from build123d import *

# Parameters (mm, degrees)
SKETCH_1_W          = 13
SKETCH_1_H          = 2.1
SKETCH_1_W_2        = 8
EXTRUDE_3_DEPTH     = 2
SKETCH_2_W          = 6.1
SKETCH_2_H          = 2.1
CUT_EXTRUDE_1_DEPTH = 2
SKETCH_12_W         = 13
SKETCH_12_H         = 2.1
EXTRUDE_9_DEPTH     = 2
SKETCH_13_R         = 1.7
EXTRUDE_10_DEPTH    = 2
SKETCH_3_W          = 16.8
SKETCH_3_H          = 2.1
EXTRUDE_4_DEPTH     = 2
SKETCH_8_R          = 1.7
CUT_EXTRUDE_4_DEPTH = 10
SKETCH_9_W          = 16.8
SKETCH_9_H          = 2.1
CUT_EXTRUDE_5_DEPTH = 10
EXTRUDE_11_DEPTH    = 2


with BuildPart() as part:
    # 草图1 → 凸台-拉伸3 (new body)
    with BuildSketch(Plane.XY):
        Polygon((0, 39.1), (0, 11.1), (8, 11.1), (21, 11.1), (29, 11.1), (29, 39.1), align=None)
        with Locations((14.5, -1.05)):
            Rectangle(SKETCH_1_W, SKETCH_1_H)
        Polygon((0, 9), (0, 0), (8, 0), (21, 0), (29, 0), (29, 9), (21, 9), (8, 9), align=None)
        with Locations((25, 10.05)):
            Rectangle(SKETCH_1_W_2, SKETCH_1_H)
        with Locations((4, 10.05)):
            Rectangle(SKETCH_1_W_2, SKETCH_1_H)
    extrude(amount=EXTRUDE_3_DEPTH)

    # 草图2 → 切除-拉伸1 (cut)
    with BuildSketch(Plane.XY.offset(2)):
        with Locations((3.05, 17.25)):
            Rectangle(SKETCH_2_W, SKETCH_2_H)
        with Locations((25.95, 17.25)):
            Rectangle(SKETCH_2_W, SKETCH_2_H)
    extrude(amount=-CUT_EXTRUDE_1_DEPTH, mode=Mode.SUBTRACT)

    # 草图12 → 凸台-拉伸9 (add)
    with BuildSketch(Plane.XY.offset(2)):
        with Locations((14.5, 10.05)):
            Rectangle(SKETCH_12_W, SKETCH_12_H)
    extrude(amount=-EXTRUDE_9_DEPTH)

    # 草图13 → 凸台-拉伸10 (add)
    with BuildSketch(Plane.XY.offset(2)):
        Polygon((8, -2.1), (0, -2.1), (0, -11.1), (8, -11.1), (8, -13.2), (21, -13.2), (21, -11.1), (29, -11.1), (29, -2.1), (21, -2.1), align=None)
        with Locations((4.5, -6.6)):
            Circle(SKETCH_13_R, mode=Mode.SUBTRACT)
        with Locations(Location((24.5, -6.6, 0), (0, 0, 180))):
            Circle(SKETCH_13_R, mode=Mode.SUBTRACT)
    extrude(amount=-EXTRUDE_10_DEPTH)

    # 草图3 → 凸台-拉伸4 (add)
    with BuildSketch(Plane.XY.offset(2)):
        with Locations((14.5, 40.15)):
            Rectangle(SKETCH_3_W, SKETCH_3_H)
    extrude(amount=-EXTRUDE_4_DEPTH)

    # 草图8 → 切除-拉伸4 (cut)
    with BuildSketch(Plane.XY.offset(2)):
        with Locations((21.5, 26.8)):
            Circle(SKETCH_8_R)
        with Locations((7.5, 26.8)):
            Circle(SKETCH_8_R)
    extrude(amount=-CUT_EXTRUDE_4_DEPTH, mode=Mode.SUBTRACT)

    # 草图9 → 切除-拉伸5 (cut)
    with BuildSketch(Plane.XY.offset(2)):
        with Locations((14.5, 40.15)):
            Rectangle(SKETCH_9_W, SKETCH_9_H)
    extrude(amount=-CUT_EXTRUDE_5_DEPTH, mode=Mode.SUBTRACT)

    # 草图11 → 凸台-拉伸11 (add)
    with BuildSketch(Plane.XY.offset(2)):
        Polygon((6.1, 39.1), (6.1, 41.2), (0, 41.2), (0, 44.2), (29, 44.2), (29, 41.2), (22.9, 41.2), (22.9, 39.1), align=None)
    extrude(amount=-EXTRUDE_11_DEPTH)


solid = part.part
Source: CAD feature listing. Evaluate the final solid. Frame: model axes, mm. A direction names the side the tool comes from. Round coordinates to 2 decimals unless told otherwise and drop trailing zeros. Loops run counter-clockwise (first coordinate to the right, second up) from the corner with the lowest first, then second, coordinate; pieces in that order, holes last. Notation, with made-up numbers: (85.5, -23.5) -> (141.5, -23.5) arc R26 ccw to (141.5, -7.5) -> close; hole circle Ø6 at (86, -3). An arc over 180 degrees is marked (long way). Answer as a JSON object with one key per item and string values. Group by question number.
Q1. Access query for faces 1 (the flat face through (6.1, 17, 1)), 2 (the flat face through (26, 39.1, 1)), 3 (the flat face through (4, -11.1, 1)). Directions: +Z, -Z, +X, -X, +Y, -Y. A direction counts if a zero-diameter tool reaches every point of the face in a straight line with its end or side. Return the directions, or none.
Q2. Section query A-A (x = 4.5). Output: boundary loops of the cut face in (y, z).
Q3. Ray query, line 1 (Y direction, x = 4.5, z = 0.7); line 2 (Y direction, x = 7.5, z = 1.35); line 3 (Y direction, x = 23, z = 0.7). Return the intervals inside material, ascending. Write a range as from..to.
Q4. Section query B-B (y = -6.6). Output: boundary loops of the cut face in (x, z).
Q5. Mould query, pull axis X, two halves, no side actions, for faces 4 (the flat face through (14, 16, 2)), 5 (the flat face through (21, -1, 1)), 6 (the cylindrical face through (6.07, -7.25, 1.01)). Classes: pulls with the +X half, pulls with the -X half, needs draft (parallel to the pull), parting line crosses it, or undercut.
Q6. Section query C-C (z = 1.25). State how many separate pieces and enclosed holes the cut face has, plus the area to 3 significant figures.
Q7. Contact query for flat-ended pins moving along their axis: P1, Ø0.6, axis at y = 40.5, z = 1, coming from the +X side; P2, Ø0.6, axis at x = 25.5, z = 1, coming from the -Y side; P3, Ø3, axis at x = 4.5, y = -6.6, coming from the +Z side. Output: stop coordinate, or through.
Completed:
{
 "1": {"face 1": "+Z, -Z, -X", "face 2": "+Z, -Z, +X", "face 3": "+Z, -Z, -X, -Y"},
 "2": {"outline": "(-11.1, 0) -> (-8.3, 0) -> (-8.3, 2) -> (-11.1, 2) -> close; (-4.9, 0) -> (-2.1, 0) -> (-2.1, 2) -> (-4.9, 2) -> close; (0, 0) -> (16.2, 0) -> (16.2, 2) -> (0, 2) -> close; (18.3, 0) -> (39.1, 0) -> (39.1, 2) -> (18.3, 2) -> close; (41.2, 0) -> (44.2, 0) -> (44.2, 2) -> (41.2, 2) -> close"},
 "3": {"line 1": "-11.1..-8.3, -4.9..-2.1, 0..16.2, 18.3..39.1, 41.2..44.2", "line 2": "-11.1..-2.1, 0..25.1, 28.5..44.2", "line 3": "-11.1..-7.4, -5.8..-2.1, 0..16.2, 18.3..26, 27.6..39.1, 41.2..44.2"},
 "4": {"outline": "(0, 0) -> (2.8, 0) -> (2.8, 2) -> (0, 2) -> close; (6.2, 0) -> (22.8, 0) -> (22.8, 2) -> (6.2, 2) -> close; (26.2, 0) -> (29, 0) -> (29, 2) -> (26.2, 2) -> close"},
 "5": {"face 4": "needs draft", "face 5": "pulls with the +X half", "face 6": "undercut"},
 "6": {"separate pieces": "1", "enclosed holes": "4", "area": "1,510 mm²"},
 "7": {"P1": "x = 22.9", "P2": "y = -11.1", "P3": "through"}
}
